Here's how the part is built. I have some questions about the finished solid (model axes, mm). Give positions to 0.01 mm unless a question says otherwise; leave off trailing zeros. Loops run counter-clockwise (first coordinate to the right, second up) from the corner with the lowest first, then second, coordinate; pieces in that order, holes last.
Q1. If we section it at A-A (x = 35): Please give me the cut outline in (y, z), plus the area to 3 significant figures.
Q2. I need wall thicknesses on line 1 (X direction, y = 1, z = 1.1); line 2 (Y direction, x = 21, z = 1.45); line 3 (X direction, y = 28, z = 0.6). Which ranges of each line are inside material? Lowest first, please.
Q3. If we section it at D-D (y = 3): Please give me the cut outline in (x, z).
Q4. If we section it at C-C (z = 4.65): Give the number of separate pieces and of enclosed holes in the cut face, plus the area to 3 significant figures.
Q5. If we section it at B-B (y = 17): Please give me the cut outline in (x, z), plus the area to 3 significant figures.
from build123d import *

# Parameters (mm, degrees)
F0_R     = 1.75
F0_W     = 100.394129
F0_H     = 41.936789
F0_R_2   = 2
F0_R_3   = 3.75
F1_DEPTH = 5.5


with BuildPart() as f1:
    # F0 (on Top) → F1 (new body)
    with BuildSketch(Plane.XY):
        Polygon((97.50326, 35.808698), (-102.59674, 35.808698), (-102.59674, -4.191302), (-96.59674, -4.191302), (-96.59674, -13.191302), (-102.59674, -13.191302), (-102.59674, -36.191302), (97.50326, -36.191302), (97.50326, -13.191302), (91.50326, -13.191302), (91.50326, -4.191302), (97.50326, -4.191302), align=None)
        with Locations((-72.59103, -21.273935)):
            Circle(F0_R, mode=Mode.SUBTRACT)
        with Locations((-12.867824, -1.88542)):
            Rectangle(F0_W, F0_H, mode=Mode.SUBTRACT)
        with Locations((71.91792, -21.28585)):
            Circle(F0_R, mode=Mode.SUBTRACT)
        with Locations((61.65615, -15.016859)):
            Circle(F0_R_2, mode=Mode.SUBTRACT)
        with Locations((-99.59674, 11.308698)):
            Circle(F0_R, mode=Mode.SUBTRACT)
        with Locations((-72.609478, 28.211436)):
            Circle(F0_R, mode=Mode.SUBTRACT)
        with Locations((62.149974, 1.143538)):
            Circle(F0_R_3, mode=Mode.SUBTRACT)
        with Locations((94.50326, 11.308698)):
            Circle(F0_R, mode=Mode.SUBTRACT)
        with Locations((71.900612, 28.217664)):
            Circle(F0_R, mode=Mode.SUBTRACT)
    extrude(amount=F1_DEPTH)


solid = f1.part
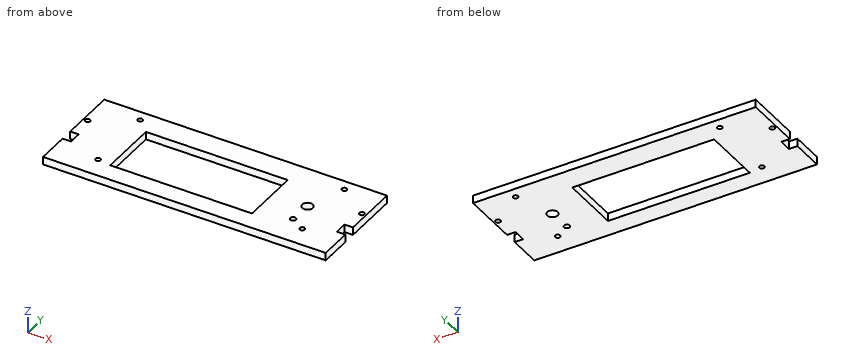
Check sheet entries:
1. outline: (-36.19, 0) - (-22.85, 0) - (-22.85, 5.5) - (-36.19, 5.5) - close; (19.08, 0) - (35.81, 0) - (35.81, 5.5) - (19.08, 5.5) - close
1. area: 165 mm2
2. line 1: x = -102.6 to -63.06, 37.33 to 58.4, 65.9 to 97.5
2. line 2: y = -36.19 to -22.85, 19.08 to 35.81
2. line 3: x = -102.6 to -74.35, -70.87 to 70.16, 73.64 to 97.5
3. outline: (-102.6, 0) - (-63.06, 0) - (-63.06, 5.5) - (-102.6, 5.5) - close; (37.33, 0) - (58.89, 0) - (58.89, 5.5) - (37.33, 5.5) - close; (65.41, 0) - (97.5, 0) - (97.5, 5.5) - (65.41, 5.5) - close
4. separate pieces: 1
4. enclosed holes: 9
4. area: 9,970 mm2
5. outline: (-102.6, 0) - (-63.06, 0) - (-63.06, 5.5) - (-102.6, 5.5) - close; (37.33, 0) - (97.5, 0) - (97.5, 5.5) - (37.33, 5.5) - close
5. area: 548 mm2
